```python
from build123d import *

# Parameters (mm, degrees)
ESBO_O1_W             = 22
ESBO_O1_H             = 55
CORTE_EXTRUS_O1_DEPTH = 20
CIRPATTERN1_COUNT     = 12
CORTE_EXTRUS_O2_DEPTH = 98.532046016
CIRPATTERN2_COUNT     = 12


with BuildPart() as part:
    # Esboço1 → Revolução1 (revolve)
    with BuildSketch(Plane.XY, mode=Mode.PRIVATE) as revolu_o1_sk:
        with Locations((11, 40)):
            Rectangle(ESBO_O1_W, ESBO_O1_H)
    revolve(revolu_o1_sk.sketch.rotate(Axis((0, 0, 0), (1, 0, 0)), 90), axis=Axis((0, 0, 0), (1, 0, 0)))

    # Esboço2 → Corte-extrusão1 (cut)
    with BuildSketch(Plane(origin=(22, 0, 0), x_dir=(0, 0, -1), z_dir=(1, 0, 0))):
        with BuildLine():
            Line((1, 57.49130369), (1, 14.465476141))
            ThreePointArc((1, 14.465476141), (4.473814272, 13.792569951), (7.681217142, 12.298329286))
            Line((7.681217142, 12.298329286), (29.184480159, 49.543073359))
            ThreePointArc((29.184480159, 49.543073359), (15.606706954, 55.34149165), (1, 57.49130369))
        make_face()
    corte_extrus_o1 = extrude(amount=-CORTE_EXTRUS_O1_DEPTH, mode=Mode.SUBTRACT)

    # CirPattern1: Corte-extrusão1 ×12 about axis
    cirpattern1_axis = Axis((0, 0, 0), (1, 0, 0))
    for i in range(1, CIRPATTERN1_COUNT):
        add(corte_extrus_o1.rotate(cirpattern1_axis, i * 360 / CIRPATTERN1_COUNT), mode=Mode.SUBTRACT)

    # Esboço3 → Corte-extrusão2 (cut, through all)
    with BuildSketch(Plane(origin=(20, 0, 0), x_dir=(0, 0, -1), z_dir=(1, 0, 0))):
        with BuildLine():
            Line((29.184480159, 49.543073359), (34.184643112, 58.203609641))
            ThreePointArc((34.184643112, 58.203609641), (18.195083867, 65.001453238), (1, 67.492592186))
            Line((1, 67.492592186), (1, 57.49130369))
            ThreePointArc((1, 57.49130369), (15.606706954, 55.34149165), (29.184480159, 49.543073359))
        make_face()
    corte_extrus_o2 = extrude(amount=-CORTE_EXTRUS_O2_DEPTH, mode=Mode.SUBTRACT)

    # CirPattern2: Corte-extrusão2 ×12 about axis
    cirpattern2_axis = Axis((0, 0, 0), (1, 0, 0))
    for i in range(1, CIRPATTERN2_COUNT):
        add(corte_extrus_o2.rotate(cirpattern2_axis, i * 360 / CIRPATTERN2_COUNT), mode=Mode.SUBTRACT)


solid = part.part
```
For this review, take the finished solid that the model builds, in its own axes (mm). A direction names the side the tool comes from. Coordinates: 2 decimals unless noted, no trailing zeros. Write each loop counter-clockwise with the first axis right and the second up, starting at its lowest first coordinate (ties: lowest second). Pieces come first, ordered by that corner, then holes.
(1) Add section B-B on y = 45.5. Give the boundary of the cut face in (x, z).
(2) Add section A-A on z = 4.5. Give the boundary of the cut face in (x, y), then the cut area to 3 significant figures.
(3) For pin 1 Ø1.5 at (y, z) = (7, -26) entering from +X; pin 2 Ø5 at (x, z) = (14.5, 16) entering from +Y; pin 3 Ø1 at (x, y) = (7.5, -3.5) entering from -Z; pin 4 Ø22.5 at (y, z) = (0, 0) entering from -X, all flat-tipped, find the tip position at first contact; note any pin that passes through.
(4) The part is to be moulded in two halves that separate along Y. For faces 1 (the face through (1.01, -55.68, -14.36)), 2 (the face through (2, 40, -12)), 3 (the face through (2, 10, -41)), say which applies: +Y half, -Y half, draft (parallel to the pull), parting line (faces both ways), or undercut.
(5) Tool access review of faces 4 (the face through (21.014, 15.806, 55.285)), 5 (the face through (1.014, -40.272, 41.042)), 6 (the face through (20, -15, 61)): name each direction out of +Z, -Z, +X, -X, +Y, -Y from which nothing blocks a thin tool from reaching the whole face with its end or side.
(6) Wall thickness on probe 1 along Y at (x, z) = (5.5, 0); probe 2 along Z at (x, y) = (19.5, 55.5); probe 3 along Z at (x, y) = (4.75, 21): over which ranges is each line inside the solid? List them lowest first.
(7) Add section C-C on y = -16.5. Count the separate pieces of the cut face and the enclosed holes in it, then the cut area to 3 significant figures.
Answer sheet:
1. outline: (0, -35.16) - (2, -35.16) - (2, -27.42) - (22, -27.42) - (22, -26.85) - (2, -26.85) - (2, -1) - (22, -1) - (22, -0.5) - (2, -0.5) - (2, 25.11) - (22, 25.11) - (22, 25.69) - (2, 25.69) - (2, 35.16) - (0, 35.16) - close; (20, -49.86) - (22, -49.86) - (22, -35.16) - (20, -35.16) - close; (20, 35.16) - (22, 35.16) - (22, 49.86) - (20, 49.86) - close
2. outline: (0, -57.32) - (2, -57.32) - (2, -13.78) - (22, -13.78) - (22, -11.66) - (0, -11.66) - close; (0, 11.66) - (22, 11.66) - (22, 13.78) - (2, 13.78) - (2, 57.32) - (0, 57.32) - close; (20, -67.35) - (22, -67.35) - (22, -57.32) - (20, -57.32) - close; (20, 57.32) - (22, 57.32) - (22, 67.35) - (20, 67.35) - close
2. area: 308 mm2
3. pin 1: stops at x = 2
3. pin 2: stops at y = 34.04
3. pin 3: stops at z = -14.19
3. pin 4: passes through
4. face 1: -Y half
4. face 2: draft
4. face 3: undercut
5. face 4: +X
5. face 5: -X
5. face 6: +Z, -X
6. probe 1: y = -14.5 to -12.5, 12.5 to 14.5
6. probe 2: z = -33.2 to -32.62, -1 to -0.5, 30.89 to 31.46
6. probe 3: z = -38.37 to -37.38, -13.28 to -12.71, -1 to -0.5, 10.97 to 11.54, 34.37 to 35.37
7. separate pieces: 3
7. enclosed holes: 0
7. area: 334 mm2
